The model under review builds one solid part; all positions refer to its coordinate system, in mm. Coordinates: 2 decimals unless noted, no trailing zeros. Write each loop counter-clockwise with the first axis right and the second up, starting at its lowest first coordinate (ties: lowest second). Pieces come first, ordered by that corner, then holes. Notation, with made-up numbers: M -19.5,65 L -7.5,65 A32 cw -7.5,92 Z; hole C -35,23 d7. An arc over 180 degrees is marked long. Answer as CSV lines item,"result". Start each with the question number.
from build123d import *

# Parameters (mm, degrees)
F0_W     = 40
F0_H     = 100
F1_DEPTH = 40
F2_DEPTH = 100
F3_DEPTH = 20.5
F4_DEPTH = 20.5
F6_DEPTH = 25


with BuildPart() as f1:
    # F0 (on Front) → F1 (new body)
    with BuildSketch(Plane.XZ):
        Rectangle(F0_W, F0_H)
    extrude(amount=F1_DEPTH)

    # F2 (add): a face of the model
    f2_faces = [f1.faces().sort_by_distance(p)[0] for p in [
        (0, -20, 50),
    ]]
    extrude(f2_faces, amount=F2_DEPTH)

    # F3 (cut): a face of the model
    f3_faces = [f1.faces().sort_by_distance(p)[0] for p in [
        (20, -20, 50),
    ]]
    extrude(f3_faces, amount=-F3_DEPTH, mode=Mode.SUBTRACT)

    # F4 (cut): a face of the model
    f4_faces = [f1.faces().sort_by_distance(p)[0] for p in [
        (-10.25, -40, 50),
    ]]
    extrude(f4_faces, amount=-F4_DEPTH, mode=Mode.SUBTRACT)

    # F5 (on face) → F6 (cut)
    with BuildSketch(Plane.YZ.offset(-0.5)):
        with BuildLine():
            ThreePointArc((-4.5432102773, 140), (-9.75, 145.2067897227), (-14.9567897227, 140))
            ThreePointArc((-14.9567897227, 140), (-9.75, 134.7932102773), (-4.5432102773, 140))
        make_face()
    extrude(amount=-F6_DEPTH, mode=Mode.SUBTRACT)


solid = f1.part
1) Mouldability with a two-part tool opening along Z and no side actions: class faces 1 (the flat face through (-10, 0, 49)), 2 (the flat face through (-10, -10, 150)), 3 (the cylindrical face through (-10.11, -12.55, 135.61)) as +Z half, -Z half, draft (parallel to the pull), parting line (faces both ways), or undercut.
2) Take a section at A-A on y = -9.75. Give the boundary of the cut face in (x, z).
3) Take a section at B-B on z = 140. Give the boundary of the cut face in (x, y).
4) Take a section at C-C on x = -8. Give the boundary of the cut face in (y, z), and give its area (3 significant figures).
5) To check wall thickness, follow line 1 (Y direction, x = -7.75, z = 140); line 2 (Z direction, x = -5.25, y = -9.75); line 3 (Z direction, x = -6.75, y = -6.5). State the ranges of each line that lie inside material, in increasing order. Write a range as [from, to].
Results:
1,face 1,"draft"
1,face 2,"+Z half"
1,face 3,"undercut"
2,outline,"M -20,-50 L -0.5,-50 L -0.5,134.79 L -20,134.79 Z; M -20,145.21 L -0.5,145.21 L -0.5,150 L -20,150 Z"
3,outline,"M -20,-19.5 L -0.5,-19.5 L -0.5,-14.96 L -20,-14.96 Z; M -20,-4.54 L -0.5,-4.54 L -0.5,0 L -20,0 Z"
4,outline,"M -19.5,-50 L 0,-50 L 0,150 L -19.5,150 Z; hole C -9.75,140 d10.41"
4,area,"3,810 mm²"
5,line 1,"y = [-19.5, -14.96], [-4.54, 0]"
5,line 2,"z = [-50, 134.79], [145.21, 150]"
5,line 3,"z = [-50, 135.93], [144.07, 150]"
